```python
from build123d import *

# Parameters (mm, degrees)
F0_R     = 9
F0_R_2   = 6
F1_DEPTH = 3


# Not quite as in the source:
# - a feature names something its author has since deleted; it is built from what else it names


with BuildPart() as f1:
    # F0 (on Top) → F1 (new body)
    with BuildSketch(Plane.XY):
        with BuildLine():
            ThreePointArc((0, 49), (-49, 0), (0, -49))
            ThreePointArc((0, -49), (34.6482322781, -34.6482322781), (49, 0))
            ThreePointArc((49, 0), (34.6482322781, 34.6482322781), (0, 49))
        make_face()
        with BuildLine():
            ThreePointArc((31.698164825, 14.8400251593), (34.1645706023, 7.601454832), (35, 0))
            ThreePointArc((35, 0), (34.1645706023, -7.601454832), (31.698164825, -14.8400251593))
            ThreePointArc((31.698164825, -14.8400251593), (32.8762182612, -15.9446587316), (33.3108891325, -17.5))
            ThreePointArc((33.3108891325, -17.5), (31.7548586928, -20.1296296144), (28.7009211933, -20.0314034121))
            ThreePointArc((28.7009211933, -20.0314034121), (17.5, -30.3108891325), (2.9972436317, -34.8714285714))
            ThreePointArc((2.9972436317, -34.8714285714), (2.9993108288, -34.9356995144), (3, -35))
            ThreePointArc((3, -35), (2.1213203436, -37.1213203436), (0, -38))
            ThreePointArc((0, -38), (-2.1663003353, -37.0753657165), (-2.9972436317, -34.8714285714))
            ThreePointArc((-2.9972436317, -34.8714285714), (-17.5, -30.3108891325), (-28.7009211933, -20.0314034121))
            ThreePointArc((-28.7009211933, -20.0314034121), (-32.9089653438, -19), (-31.698164825, -14.8400251593))
            ThreePointArc((-31.698164825, -14.8400251593), (-35, 0), (-31.698164825, 14.8400251593))
            ThreePointArc((-31.698164825, 14.8400251593), (-32.9089653438, 19), (-28.7009211933, 20.0314034121))
            ThreePointArc((-28.7009211933, 20.0314034121), (-17.5, 30.3108891325), (-2.9972436317, 34.8714285714))
            ThreePointArc((-2.9972436317, 34.8714285714), (-0.0643004856, 37.9993108288), (3, 35))
            ThreePointArc((3, 35), (2.9993108288, 34.9356995144), (2.9972436317, 34.8714285714))
            ThreePointArc((2.9972436317, 34.8714285714), (17.5, 30.3108891325), (28.7009211933, 20.0314034121))
            ThreePointArc((28.7009211933, 20.0314034121), (31.7548586928, 20.1296296144), (33.3108891325, 17.5))
            ThreePointArc((33.3108891325, 17.5), (32.8762182612, 15.9446587316), (31.698164825, 14.8400251593))
        make_face(mode=Mode.SUBTRACT)
        with BuildLine():
            ThreePointArc((31.698164825, -14.8400251593), (34.1645706023, -7.601454832), (35, 0))
            ThreePointArc((35, 0), (34.1645706023, 7.601454832), (31.698164825, 14.8400251593))
            ThreePointArc((31.698164825, 14.8400251593), (27.7128129211, 16), (28.7009211933, 20.0314034121))
            ThreePointArc((28.7009211933, 20.0314034121), (17.5, 30.3108891325), (2.9972436317, 34.8714285714))
            ThreePointArc((2.9972436317, 34.8714285714), (0, 32), (-2.9972436317, 34.8714285714))
            ThreePointArc((-2.9972436317, 34.8714285714), (-17.5, 30.3108891325), (-28.7009211933, 20.0314034121))
            ThreePointArc((-28.7009211933, 20.0314034121), (-27.6812595181, 18.9439695603), (-27.3108891325, 17.5))
            ThreePointArc((-27.3108891325, 17.5), (-28.755547864, 14.9346708713), (-31.698164825, 14.8400251593))
            ThreePointArc((-31.698164825, 14.8400251593), (-35, 0), (-31.698164825, -14.8400251593))
            ThreePointArc((-31.698164825, -14.8400251593), (-28.755547864, -14.9346708713), (-27.3108891325, -17.5))
            ThreePointArc((-27.3108891325, -17.5), (-27.6812595181, -18.9439695603), (-28.7009211933, -20.0314034121))
            ThreePointArc((-28.7009211933, -20.0314034121), (-17.5, -30.3108891325), (-2.9972436317, -34.8714285714))
            ThreePointArc((-2.9972436317, -34.8714285714), (-2.0753657165, -32.8336996647), (0, -32))
            ThreePointArc((0, -32), (2.0753657165, -32.8336996647), (2.9972436317, -34.8714285714))
            ThreePointArc((2.9972436317, -34.8714285714), (17.5, -30.3108891325), (28.7009211933, -20.0314034121))
            ThreePointArc((28.7009211933, -20.0314034121), (27.7128129211, -16), (31.698164825, -14.8400251593))
        make_face()
        with BuildLine():
            ThreePointArc((28, 0), (19.7989898732, -19.7989898732), (0, -28))
            ThreePointArc((0, -28), (-19.7989898732, 19.7989898732), (28, 0))
        make_face(mode=Mode.SUBTRACT)
        with BuildLine():
            Line((0, -70), (0, -49))
            ThreePointArc((0, -49), (-49, 0), (0, 49))
            Line((0, 49), (-51, 49))
            ThreePointArc((-51, 49), (-61.6066017178, 44.6066017178), (-66, 34))
            Line((-66, 34), (-66, -40.2424365873))
            ThreePointArc((-66, -40.2424365873), (-64.6762407754, -46.4036408731), (-60.938608233, -51.4773850246))
            Line((-60.938608233, -51.4773850246), (-44.2561452447, -66.2349484374))
            ThreePointArc((-44.2561452447, -66.2349484374), (-39.6314702743, -69.0271919243), (-34.3175370117, -70))
            Line((-34.3175370117, -70), (0, -70))
        make_face()
        with Locations((-35, -54)):
            Circle(F0_R, mode=Mode.SUBTRACT)
        with Locations((-52, -39)):
            Circle(F0_R, mode=Mode.SUBTRACT)
        with Locations((-52, 35)):
            Circle(F0_R, mode=Mode.SUBTRACT)
        with BuildLine():
            ThreePointArc((49, 0), (34.6482322781, -34.6482322781), (0, -49))
            Line((0, -49), (0, -70))
            Line((0, -70), (34.3175370117, -70))
            ThreePointArc((34.3175370117, -70), (39.6314702743, -69.0271919243), (44.2561452447, -66.2349484374))
            Line((44.2561452447, -66.2349484374), (60.938608233, -51.4773850246))
            ThreePointArc((60.938608233, -51.4773850246), (64.6762407754, -46.4036408731), (66, -40.2424365873))
            Line((66, -40.2424365873), (66, 34))
            ThreePointArc((66, 34), (61.6066017178, 44.6066017178), (51, 49))
            Line((51, 49), (0, 49))
            ThreePointArc((0, 49), (34.6482322781, 34.6482322781), (49, 0))
        make_face()
        with Locations((35, -54)):
            Circle(F0_R, mode=Mode.SUBTRACT)
        with Locations((52, -39)):
            Circle(F0_R, mode=Mode.SUBTRACT)
        with Locations((52, 35)):
            Circle(F0_R, mode=Mode.SUBTRACT)
        with Locations((-52, 35)):
            Circle(F0_R)
        with Locations((-52, 35)):
            Circle(F0_R_2, mode=Mode.SUBTRACT)
        with Locations((-52, -39)):
            Circle(F0_R)
        with Locations((-52, -39)):
            Circle(F0_R_2, mode=Mode.SUBTRACT)
        with Locations((-35, -54)):
            Circle(F0_R)
        with Locations((-35, -54)):
            Circle(F0_R_2, mode=Mode.SUBTRACT)
        with Locations((35, -54)):
            Circle(F0_R)
        with Locations((35, -54)):
            Circle(F0_R_2, mode=Mode.SUBTRACT)
        with Locations((52, -39)):
            Circle(F0_R)
        with Locations((52, -39)):
            Circle(F0_R_2, mode=Mode.SUBTRACT)
        with Locations((52, 35)):
            Circle(F0_R)
        with Locations((52, 35)):
            Circle(F0_R_2, mode=Mode.SUBTRACT)
    extrude(amount=F1_DEPTH)


solid = f1.part
```
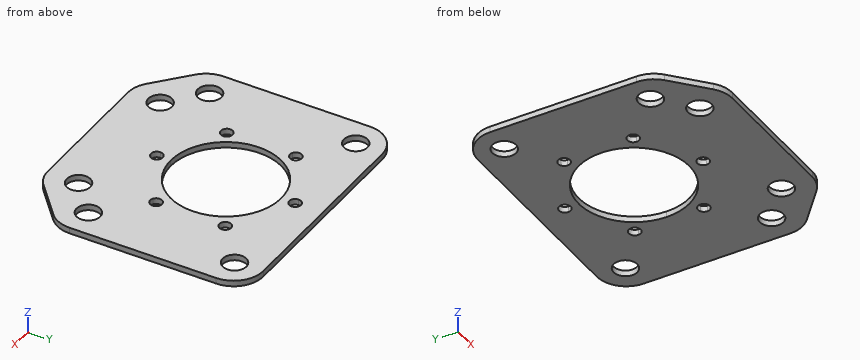
Part model, mm, in its own coordinate system. Coordinates: 2 decimals unless noted, no trailing zeros. Loops run counter-clockwise (first coordinate to the right, second up) from the corner with the lowest first, then second, coordinate; pieces in that order, holes last. Notation, with made-up numbers: (79, 42.5) - (137, 42.5) arc R21 ccw to (137, 52.5) - close; hole circle Ø2 at (58.25, 67.25). An arc over 180 degrees is marked (long way). Write item = value, one per line. Start each with the question number.
Item 1: Cut at C-C, the plane x = 14. Give the cut face in (y, z).
Item 2: Cut at D-D, the plane x = -48. Give the cut face in (y, z).
Item 3: Wall check: L1, parallel to Y at x = 35, z = 0.85; L2, parallel to X at y = 29.5, z = 1.3; L3, parallel to Y at x = -53.5, z = 2.2. Give the ranges that are in metal, low to high. Write a range as from..to.
Item 4: Cut at B-B, the plane y = -2. Give the cut face in (x, z).
Item 5: Flat gauge pin, fed straight in: pin 1 Ø14 at (x, y) = (52, -39) entering from +Z. Where does the tip first touch, or does it go through?
Item 6: Cut at A-A, the plane y = -54. Give the cut face in (x, z).
The answers:
q1.outline = (-70, 0) - (-24.25, 0) - (-24.25, 3) - (-70, 3) - close; (24.25, 0) - (49, 0) - (49, 3) - (24.25, 3) - close
q2.outline = (-62.92, 0) - (-43.47, 0) - (-43.47, 3) - (-62.92, 3) - close; (-34.53, 0) - (30.53, 0) - (30.53, 3) - (-34.53, 3) - close; (39.47, 0) - (49, 0) - (49, 3) - (39.47, 3) - close
q3.L1 = -69.98..-60, -48..49
q3.L2 = -66..-54.4, -49.6..49.6, 54.4..66
q3.L3 = -58.06..-44.81, -33.19..29.19, 40.81..48.79
q4.outline = (-66, 0) - (-27.93, 0) - (-27.93, 3) - (-66, 3) - close; (27.93, 0) - (66, 0) - (66, 3) - (27.93, 3) - close
q5.pin_1 = 3
q6.outline = (-58.09, 0) - (-41, 0) - (-41, 3) - (-58.09, 3) - close; (-29, 0) - (29, 0) - (29, 3) - (-29, 3) - close; (41, 0) - (58.09, 0) - (58.09, 3) - (41, 3) - close
